Here's how the part is built. I have some questions about the finished solid (model axes, mm). Face numbers are marked on the shaded views. A direction names the side the tool comes from. Round coordinates to 2 decimals unless told otherwise and drop trailing zeros. Loops run counter-clockwise (first coordinate to the right, second up) from the corner with the lowest first, then second, coordinate; pieces in that order, holes last. Notation, with made-up numbers: M -22,-39 L 2,-39 A21 ccw 2,-9 Z; hole C 9.5,17 d10. An arc over 180 degrees is marked long. Write each question's results on one line, items separated by ' | '. Start each with the question number.
```python
from build123d import *

# Parameters (mm, degrees)
BOSS_EXTRUDE1_DEPTH      = 47.99
BOSS_EXTRUDE1_DEPTH_BACK = 47.99
SKETCH2_R                = 5.35
BOSS_EXTRUDE2_DEPTH      = 33.56
BOSS_EXTRUDE2_DEPTH_BACK = 33.56
SKETCH3_R                = 8.89
CHAMFER1_SIZE            = 4.399409051
CHAMFER1_SIZE_2          = 2.54


with BuildPart() as part:
    # Sketch2 → Boss-Extrude1 (new, two sides: drawn at the far end of the back side and taken through both)
    with BuildSketch(Plane.XY.offset(-BOSS_EXTRUDE1_DEPTH_BACK)):
        with Locations(Location((0, 160.02, 0), (0, 0, 180))):
            Circle(SKETCH2_R)
    extrude(amount=BOSS_EXTRUDE1_DEPTH + BOSS_EXTRUDE1_DEPTH_BACK)

    # Sketch3 → Boss-Extrude2 (add, two sides: drawn at the far end of the back side and taken through both)
    with BuildSketch(Plane.XY.offset(-BOSS_EXTRUDE2_DEPTH_BACK)):
        with Locations(Location((0, 160.02, 0), (0, 0, 180))):
            Circle(SKETCH3_R)
    extrude(amount=BOSS_EXTRUDE2_DEPTH + BOSS_EXTRUDE2_DEPTH_BACK)

    # Chamfer1
    # the kernel refuses this chamfer: 4.399409051, 2.54 mm, written as the material it takes off along each edge
    with BuildSketch(Plane(origin=(0, 160.02, -33.56), x_dir=(-1, 0, 0), z_dir=(0, 1, 0))) as chamfer1_piece_1:
        Polygon((8.89, CHAMFER1_SIZE), (8.89 - CHAMFER1_SIZE_2, 0), (8.89, 0), align=None)
    revolve(axis=Axis((0, 160.02, -33.56), (0, 0, 1)), mode=Mode.SUBTRACT)
    with BuildSketch(Plane(origin=(0, 160.02, 33.56), x_dir=(-1, 0, 0), z_dir=(0, 1, 0))) as chamfer1_piece_2_section:
        Polygon((8.89 - CHAMFER1_SIZE, 0), (8.89, -CHAMFER1_SIZE_2), (8.89, 0), align=None)
    chamfer1_piece_2 = revolve(axis=Axis((0, 160.02, 33.56), (0, 0, 1)), mode=Mode.PRIVATE)
    chamfer1_piece_2 = chamfer1_piece_2 - Plane(origin=(0, 160.02, 32.054862078), x_dir=(-1, 0, 0), z_dir=(0, 0, -1)) * Cylinder(5.35, 36, mode=Mode.PRIVATE)
    add(chamfer1_piece_2, mode=Mode.SUBTRACT)


solid = part.part
```
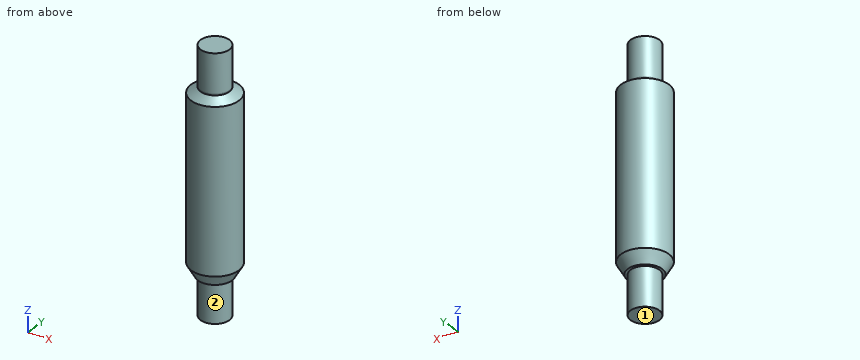
1. Which directions (+Z, -Z, +X, -X, +Y, -Y) give clear straight access to the entire face, cutting with the end or side of a thin tool? Please do the marked faces 1 and 2.
2. I need wall thicknesses on line 1 along Z through (x, y) = (-2.5, 155.25); line 2 along Z through (x, y) = (-4.25, 164.5); line 3 along Y through (x, z) = (-3, -9). Which ranges of each line are inside material? Lowest first, please.
3. I want a section at C-C on z = 9. List the corners of the cut face in (x, y) for me.
4. I want a section at A-A on x = 0. List the corners of the cut face in (y, z) for me, plus the area to 3 significant figures.
5. For pin 1 (4 mm diameter, centred on y = 162.5, z = -28.5, fed in from +X); pin 2 (8 mm diameter, centred on x = 5, z = -16.5, fed in from -Y); pin 3 (1.5 mm diameter, centred on y = 159, z = 37.5, fed in from +X), each with a flat end and sliding along its axis, tell me the tip position at first contact or that it passes through.
6. I want a section at B-B on y = 160.02. List the corners of the cut face in (x, z) for me.
Outcome:
1) face 1: -Z, +X, -X, +Y, -Y | face 2: -Z
2) line 1: -33.56 to 33.04 | line 2: -33.56 to 32.59 | line 3: 151.65 to 168.39
3) outline: C 0,160.02 d17.78
4) outline: M 151.13,-29.16 L 153.67,-33.56 L 154.67,-33.56 L 154.67,-47.99 L 165.37,-47.99 L 165.37,-33.56 L 166.37,-33.56 L 168.91,-29.16 L 168.91,31.02 L 165.37,33.06 L 165.37,47.99 L 154.67,47.99 L 154.67,33.06 L 151.13,31.02 Z | area: 1,480 mm2
5) pin 1: x = 8.88 | pin 2: y = 151.19 | pin 3: x = 5.34
6) outline: M -8.89,-29.16 L -6.35,-33.56 L -5.35,-33.56 L -5.35,-47.99 L 5.35,-47.99 L 5.35,-33.56 L 6.35,-33.56 L 8.89,-29.16 L 8.89,31.02 L 5.35,33.06 L 5.35,47.99 L -5.35,47.99 L -5.35,33.06 L -8.89,31.02 Z
